Verification items for the finished model (mm, model axes). Face numbers are marked on the shaded views. A direction names the side the tool comes from. Give positions to 0.01 mm unless a question says otherwise; leave off trailing zeros. Order: outer loops, then holes, each group sorted by start corner. A loop starts at its lowest first (then second) coordinate and runs counter-clockwise, first axis right, second up.
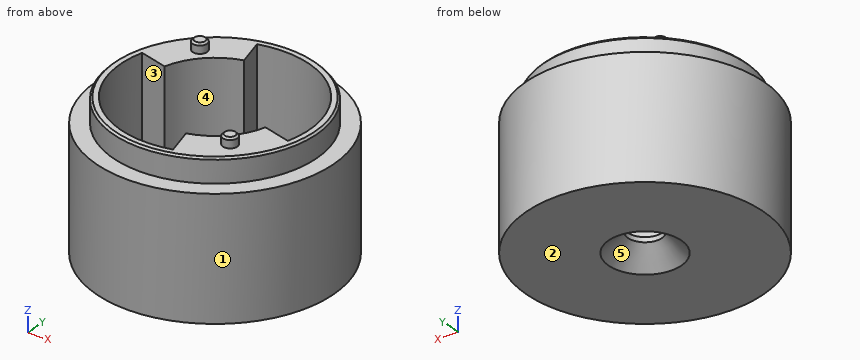
from build123d import *

# Parameters (mm, degrees)
SKETCH005_R           = 12.25
SKETCH005_R_2         = 1.75
PAD004_DEPTH          = 2.5
CHAMFER001_SIZE       = 2
PAD005_DEPTH          = 12.5
POLARPATTERN001_COUNT = 2
SKETCH008_R           = 0.75
PAD006_DEPTH          = 1
POLARPATTERN002_COUNT = 2
CHAMFER002_SIZE       = 0.2


with BuildPart() as part:
    # Sketch005 → Pad004 (new body)
    with BuildSketch(Plane.XY):
        Circle(SKETCH005_R)
        Circle(SKETCH005_R_2, mode=Mode.SUBTRACT)
    extrude(amount=-PAD004_DEPTH)

    # Chamfer001
    chamfer001_edges = [part.edges().sort_by_distance(p)[0] for p in [
        (-1.75, 0, -2.5),
    ]]
    chamfer(chamfer001_edges, length=CHAMFER001_SIZE)

    # Sketch006 → Revolution (revolve)
    with BuildSketch(Plane.XZ):
        Polygon((12.25, 0), (12.25, 10), (10.5, 10), (10.5, 12.5), (9.75, 12.5), (9.75, 0), align=None)
    revolve(axis=Axis((0, 0, 0), (0, 0, 1)))

    # Sketch007 → Pad005 (join)
    with BuildSketch(Plane.XY):
        with BuildLine():
            ThreePointArc((-2.523486, 9.417777), (-6.894291, 6.894291), (-9.417777, 2.523486))
            Line((-6.519999, 1.747029), (-9.417777, 2.523486))
            ThreePointArc((-1.747029, 6.519999), (-4.772971, 4.772971), (-6.519999, 1.747029))
            Line((-2.523486, 9.417777), (-1.747029, 6.519999))
        make_face()
    pad005 = extrude(amount=PAD005_DEPTH)

    # PolarPattern001: Pad005 ×2 about axis
    polarpattern001_axis = Axis((0, 0, 0), (0, 0, 1))
    for i in range(1, POLARPATTERN001_COUNT):
        add(pad005.rotate(polarpattern001_axis, i * 360 / POLARPATTERN001_COUNT))

    # Sketch008 (on DatumPlane) → Pad006 (join)
    with BuildSketch(Plane.XY.offset(12.5)):
        with Locations((-5.833631, 5.833631)):
            Circle(SKETCH008_R)
    pad006 = extrude(amount=PAD006_DEPTH)

    # PolarPattern002: Pad006 ×2 about axis
    polarpattern002_axis = Axis((0, 0, 12.5), (0, 0, 1))
    for i in range(1, POLARPATTERN002_COUNT):
        add(pad006.rotate(polarpattern002_axis, i * 360 / POLARPATTERN002_COUNT))

    # Chamfer002
    chamfer002_edges = [part.edges().sort_by_distance(p)[0] for p in [
        (-6.583631, 5.833631, 13.5),
        (6.583631, -5.833631, 13.5),
        (-10.5, 0, 12.5),
    ]]
    chamfer(chamfer002_edges, length=CHAMFER002_SIZE)


solid = part.part
(1) Section check A-A, the plane x = 0. Enter the section's corners in (y, z), then the cut area to 3 significant figures.
Solved:
outline: (-12.25, -2.5) - (-3.75, -2.5) - (-1.75, -0.5) - (-1.75, 0) - (-9.75, 0) - (-9.75, 12.5) - (-10.3, 12.5) - (-10.5, 12.3) - (-10.5, 10) - (-12.25, 10) - close; (1.75, -0.5) - (3.75, -2.5) - (12.25, -2.5) - (12.25, 10) - (10.5, 10) - (10.5, 12.3) - (10.3, 12.5) - (9.75, 12.5) - (9.75, 0) - (1.75, 0) - close
area: 102 mm2
(2) Section check B-B, the plane z = 11.5. Enter the section's corners in (x, y), then the cut area to 3 significant figures.
Solved:
outline: circle Ø21 at (0, 0); hole (-9.42, 2.52) arc R9.75 ccw to (2.52, -9.42) - (1.75, -6.52) arc R6.75 ccw to (6.52, -1.75) - (9.42, -2.52) arc R9.75 ccw to (-2.52, 9.42) - (-1.75, 6.52) arc R6.75 ccw to (-6.52, 1.75) - close
area: 99.5 mm2
(3) Section check D-D, the plane z = 6.5. Enter the section's corners in (x, y).
Solved:
outline: circle Ø24.5 at (0, 0); hole (-9.42, 2.52) arc R9.75 ccw to (2.52, -9.42) - (1.75, -6.52) arc R6.75 ccw to (6.52, -1.75) - (9.42, -2.52) arc R9.75 ccw to (-2.52, 9.42) - (-1.75, 6.52) arc R6.75 ccw to (-6.52, 1.75) - close
(4) Scan lines: line 1 (Y direction, x = 0, z = -0.2); line 2 (Z direction, x = -6.25, y = -4.5); line 3 (Y direction, x = 4.25, z = 4.75). Record each from-to range of solid material in increasing order.
Solved:
line 1: y = -12.25 to -1.75, 1.75 to 12.25
line 2: z = -2.5 to 0
line 3: y = -11.49 to -5.24, 8.77 to 11.49
(5) Set-up check for the marked faces 4 and 5: record each of +Z, -Z, +X, -X, +Y, -Y from which the full face is reachable in a straight line by a thin tool's end or side.
Solved:
face 4: +Z
face 5: -Z
(6) Go/stop test with flat-tipped pins: pin 1 (1 mm diameter, centred on x = -2, z = 3, fed in from -Y); pin 2 (3 mm diameter, centred on x = 4.5, z = 5, fed in from +Y); pin 3 (4.5 mm diameter, centred on x = 0, y = 0, fed in from -Z). Record where each tip stops, or that it passes through.
Solved:
pin 1: stops at y = -12.16
pin 2: stops at y = 11.88
pin 3: stops at z = -1
(7) Release check for a two-part mould opening along X. For the marked faces 1, 2 and 3 record: pulls with the +X half, pulls with the -X half, needs draft (parallel to the pull), parting line crosses it, or undercut.
Solved:
face 1: parting line crosses it
face 2: needs draft
face 3: undercut
